Work out the finished part from the listing and answer in its coordinate system (mm). Face numbers are marked on the shaded views. A direction names the side the tool comes from. Round coordinates to 2 decimals unless told otherwise and drop trailing zeros. Loops run counter-clockwise (first coordinate to the right, second up) from the corner with the lowest first, then second, coordinate; pieces in that order, holes last. Notation, with made-up numbers: (-5, 41.25) - (18, 41.25) arc R13 cw to (18, 59.25) - close; hole circle Ø1 at (35.25, 18). An arc over 180 degrees is marked (long way). Return JSON: item names as keys, results as strings.
Autodesk Inventor part; units mm, degrees
ref_plane "YZ Plane" through (0, 0, 0) normal (1, 0, 0) x (0, 1, 0)
ref_plane "XZ Plane" through (0, 0, 0) normal (0, 1, 0) x (-1, 0, 0)
ref_plane "XY Plane" through (0, 0, 0) normal (0, 0, 1) x (1, 0, 0)
sketch "스케치1" plane through (0, 0, 0) normal (1, 0, 0) x (0, 1, 0)
  line L0 (0, 0) -> (0, -35)
  line L1 (0, -35) -> (-28, -35)
  line L2 (-28, -35) -> (-28, 0)
  line L3 (-28, 0) -> (0, 0)
  line L4 (0, -23) -> (-28, -23)
  line L5 (-28, -23) -> (-28, -27.5)
  line L6 (-28, -27.5) -> (0, -27.5)
  line L7 (0, -27.5) -> (0, -23)
  point P0 (0, -27.5)
  dimension "d0" = 35
  dimension "d1" = 28
  dimension "d2" = 7.5
  dimension "d3" = 4.5
extrude "돌출1" add sketch "스케치1" along normal blind 5 contours L0 L1 L2 L6
extrude "돌출2" add sketch "스케치1" along normal blind 35 contours L0 L6 L2 L4
extrude "돌출3" add sketch "스케치1" along normal blind 5 contours L0 L4 L2 L3
sketch "스케치2" plane through (5, 0, 0) normal (1, 0, 0) x (0, 0, -1)
  point P0 (0, 0)
sketch "스케치3" plane through (0, -28, -35) normal (0, -1, 0) x (1, 0, 0)
  line L0 (0, 35) -> (5, 35)
  arc A0 (6.5, 34.523) -> (5, 35) centre (5, 32.403) ccw
  arc A1 (5, 33.546) -> (6.5, 34.023) centre (5, 36.143) ccw
  line L1 (5, 35) -> (9.1174, 35) construction
  line L2 (5, 33.546) -> (9.1174, 33.546) construction
  line L3 (5, 35) -> (5, 12) construction
  line L4 (6.5, 34.523) -> (6.5, 34.023)
  line L5 (5, 35) -> (5, 33.546)
  arc A2 (6.5, 32.342) -> (5, 32.819) centre (5, 30.222) ccw
  arc A3 (5, 31.365) -> (6.5, 31.842) centre (5, 33.962) ccw
  line L6 (5, 32.819) -> (9.1174, 32.819) construction
  line L7 (5, 31.365) -> (9.1174, 31.365) construction
  line L8 (6.5, 32.342) -> (6.5, 31.842)
  line L9 (5, 32.819) -> (5, 31.365)
  arc A4 (6.5, 30.161) -> (5, 30.638) centre (5, 28.041) ccw
  arc A5 (5, 29.184) -> (6.5, 29.661) centre (5, 31.781) ccw
  line L10 (5, 30.638) -> (9.1174, 30.638) construction
  line L11 (5, 29.184) -> (9.1174, 29.184) construction
  line L12 (6.5, 30.161) -> (6.5, 29.661)
  line L13 (5, 30.638) -> (5, 29.184)
  arc A6 (6.5, 27.98) -> (5, 28.457) centre (5, 25.86) ccw
  arc A7 (5, 27.003) -> (6.5, 27.48) centre (5, 29.6) ccw
  line L14 (5, 28.457) -> (9.1174, 28.457) construction
  line L15 (5, 27.003) -> (9.1174, 27.003) construction
  line L16 (6.5, 27.98) -> (6.5, 27.48)
  line L17 (5, 28.457) -> (5, 27.003)
  arc A8 (6.5, 25.799) -> (5, 26.276) centre (5, 23.679) ccw
  arc A9 (5, 24.822) -> (6.5, 25.299) centre (5, 27.419) ccw
  line L18 (5, 26.276) -> (9.1174, 26.276) construction
  line L19 (5, 24.822) -> (9.1174, 24.822) construction
  line L20 (6.5, 25.799) -> (6.5, 25.299)
  line L21 (5, 26.276) -> (5, 24.822)
  arc A10 (6.5, 23.618) -> (5, 24.095) centre (5, 21.498) ccw
  arc A11 (5, 22.641) -> (6.5, 23.118) centre (5, 25.238) ccw
  line L22 (5, 24.095) -> (9.1174, 24.095) construction
  line L23 (5, 22.641) -> (9.1174, 22.641) construction
  line L24 (6.5, 23.618) -> (6.5, 23.118)
  line L25 (5, 24.095) -> (5, 22.641)
  arc A12 (6.5, 21.437) -> (5, 21.914) centre (5, 19.317) ccw
  arc A13 (5, 20.46) -> (6.5, 20.937) centre (5, 23.057) ccw
  line L26 (5, 21.914) -> (9.1174, 21.914) construction
  line L27 (5, 20.46) -> (9.1174, 20.46) construction
  line L28 (6.5, 21.437) -> (6.5, 20.937)
  line L29 (5, 21.914) -> (5, 20.46)
  arc A14 (6.5, 19.256) -> (5, 19.733) centre (5, 17.136) ccw
  arc A15 (5, 18.279) -> (6.5, 18.756) centre (5, 20.876) ccw
  line L30 (5, 19.733) -> (9.1174, 19.733) construction
  line L31 (5, 18.279) -> (9.1174, 18.279) construction
  line L32 (6.5, 19.256) -> (6.5, 18.756)
  line L33 (5, 19.733) -> (5, 18.279)
  arc A16 (6.5, 17.075) -> (5, 17.552) centre (5, 14.955) ccw
  arc A17 (5, 16.098) -> (6.5, 16.575) centre (5, 18.695) ccw
  line L34 (5, 17.552) -> (9.1174, 17.552) construction
  line L35 (5, 16.098) -> (9.1174, 16.098) construction
  line L36 (6.5, 17.075) -> (6.5, 16.575)
  line L37 (5, 17.552) -> (5, 16.098)
  arc A18 (6.5, 14.894) -> (5, 15.371) centre (5, 12.774) ccw
  arc A19 (5, 13.917) -> (6.5, 14.394) centre (5, 16.514) ccw
  line L38 (5, 15.371) -> (9.1174, 15.371) construction
  line L39 (5, 13.917) -> (9.1174, 13.917) construction
  line L40 (6.5, 14.894) -> (6.5, 14.394)
  line L41 (5, 15.371) -> (5, 13.917)
  arc A20 (6.5, 12.713) -> (5, 13.19) centre (5, 10.593) ccw
  arc A21 (5, 11.736) -> (6.5, 12.213) centre (5, 14.333) ccw
  line L42 (5, 13.19) -> (9.1174, 13.19) construction
  line L43 (5, 11.736) -> (9.1174, 11.736) construction
  line L44 (6.5, 12.713) -> (6.5, 12.213)
  line L45 (5, 13.19) -> (5, 11.736)
  point P0 (6.5, 34.273)
  point P1 (5, 34.273)
  point P2 (6.5, 32.092)
  point P3 (5, 32.092)
  point P4 (6.5, 29.911)
  point P5 (5, 29.911)
  point P6 (6.5, 27.73)
  point P7 (5, 27.73)
  point P8 (6.5, 25.549)
  point P9 (5, 25.549)
  point P10 (6.5, 23.368)
  point P11 (5, 23.368)
  point P12 (6.5, 21.187)
  point P13 (5, 21.187)
  point P14 (6.5, 19.006)
  point P15 (5, 19.006)
  point P16 (6.5, 16.825)
  point P17 (5, 16.825)
  point P18 (6.5, 14.644)
  point P19 (5, 14.644)
  point P20 (6.5, 12.463)
  point P21 (5, 12.463)
  dimension "d10" = 1.454
  dimension "d11" = 0.5
  dimension "d12" = 1.5
  dimension "d15" = 2.181
extrude "돌출4" add sketch "스케치3" against normal up to surface (28 mm away)
properties part number "stopper"
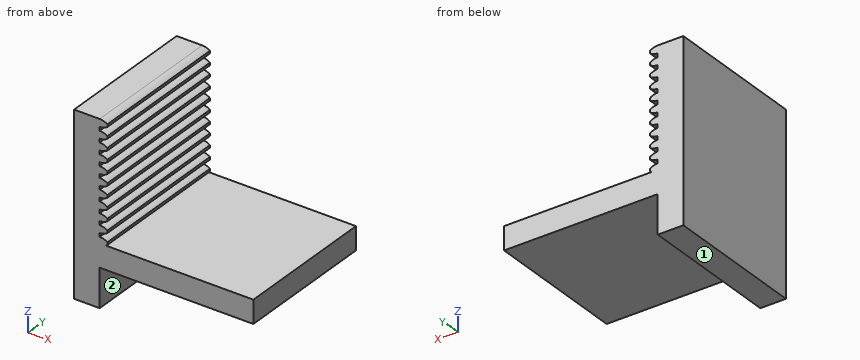
1) Flat-ended cylindrical pins translate along their axes: pin 1 (0.6 mm diameter, centred on y = -17, z = -20.5, fed in from +X); pin 2 (2 mm diameter, centred on y = -20, z = -32, fed in from +X); pin 3 (1 mm diameter, centred on x = 17, y = -12, fed in from -Z). Find the tip coordinate at first contact, or state that the pin passes through.
Verdict:
{"pin 1": "stops at x = 6.5", "pin 2": "stops at x = 5", "pin 3": "stops at z = -27.5"}
2) Section B-B (x = 32) is taken. Give the vertices of the cut face in (y, z).
Verdict:
{"outline": "(-28, -27.5) - (0, -27.5) - (0, -23) - (-28, -23) - close"}
3) A tool of negligible diameter and unlimited length cuts with its end or side. For the marked faces 1 and 2, from which of +Z, -Z, +X, -X, +Y, -Y can it reach the whole face along a straight path? Write none if from no direction.
Verdict:
{"face 1": "-Z, +X, -X, +Y, -Y", "face 2": "-Z, +X, +Y, -Y"}
4) Find the intervals of material crossed by L1, parallel to Z at x = 8, y = -24.75; L2, parallel to X at y = -2.5, z = -6; L3, parallel to X at y = -20.75, z = -14, in increasing order.
Verdict:
{"L1": "z = -27.5 to -23", "L2": "x = 0 to 5", "L3": "x = 0 to 6.5"}
5) Section A-A (z = -29) is taken. Give the vertices of the cut face in (x, y).
Verdict:
{"outline": "(0, -28) - (5, -28) - (5, 0) - (0, 0) - close"}
